```python
from build123d import *

# Parameters (mm, degrees)
F0_R     = 5.2
F0_R_2   = 2.5
F0_R_3   = 1.25
F0_R_4   = 3
F0_R_5   = 13
F1_DEPTH = 10
F2_DEPTH = 4


with BuildPart() as f1:
    # F0 (on Top) → F1 (new body)
    with BuildSketch(Plane.XY):
        with BuildLine():
            Line((-231, -59.5), (231, -59.5))
            ThreePointArc((231, -59.5), (235.242641, -57.742641), (237, -53.5))
            Line((237, -53.5), (237, 53.5))
            ThreePointArc((237, 53.5), (235.242641, 57.742641), (231, 59.5))
            Line((231, 59.5), (-231, 59.5))
            ThreePointArc((-231, 59.5), (-235.242641, 57.742641), (-237, 53.5))
            Line((-237, 53.5), (-237, -53.5))
            ThreePointArc((-237, -53.5), (-235.242641, -57.742641), (-231, -59.5))
        make_face()
        with Locations((-217, -39.5)):
            Circle(F0_R, mode=Mode.SUBTRACT)
        with Locations((-81, -13.5)):
            Circle(F0_R_2, mode=Mode.SUBTRACT)
        with Locations((-66, -13.5)):
            Circle(F0_R_2, mode=Mode.SUBTRACT)
        with Locations((-81, -4)):
            Circle(F0_R_3, mode=Mode.SUBTRACT)
        with Locations((-53, -13.5)):
            Circle(F0_R_4, mode=Mode.SUBTRACT)
        with Locations((0, -13.5)):
            Circle(F0_R_5, mode=Mode.SUBTRACT)
        with Locations((217, -39.5)):
            Circle(F0_R, mode=Mode.SUBTRACT)
        with Locations((29, -13.5)):
            Circle(F0_R_2, mode=Mode.SUBTRACT)
        with Locations((42, -13.5)):
            Circle(F0_R_2, mode=Mode.SUBTRACT)
        with Locations((55, -13.5)):
            Circle(F0_R_2, mode=Mode.SUBTRACT)
        with Locations((68, -13.5)):
            Circle(F0_R_2, mode=Mode.SUBTRACT)
        with Locations((81, -13.5)):
            Circle(F0_R_2, mode=Mode.SUBTRACT)
        with BuildLine():
            ThreePointArc((-198, 31.5), (-196.828427, 34.328427), (-194, 35.5))
            Line((-194, 35.5), (-115, 35.5))
            ThreePointArc((-115, 35.5), (-112.171573, 34.328427), (-111, 31.5))
            Line((-111, 31.5), (-111, -23.5))
            ThreePointArc((-111, -23.5), (-112.171573, -26.328427), (-115, -27.5))
            Line((-115, -27.5), (-194, -27.5))
            ThreePointArc((-194, -27.5), (-196.828427, -26.328427), (-198, -23.5))
            Line((-198, -23.5), (-198, 31.5))
        make_face(mode=Mode.SUBTRACT)
        with BuildLine():
            Line((-79, 35.5), (79, 35.5))
            ThreePointArc((79, 35.5), (81.828427, 34.328427), (83, 31.5))
            Line((83, 31.5), (83, 9.5))
            ThreePointArc((83, 9.5), (81.828427, 6.671573), (79, 5.5))
            Line((79, 5.5), (-79, 5.5))
            ThreePointArc((-79, 5.5), (-81.828427, 6.671573), (-83, 9.5))
            Line((-83, 9.5), (-83, 31.5))
            ThreePointArc((-83, 31.5), (-81.828427, 34.328427), (-79, 35.5))
        make_face(mode=Mode.SUBTRACT)
        with Locations((-217, 39.5)):
            Circle(F0_R, mode=Mode.SUBTRACT)
        with BuildLine():
            Line((111, -23.5), (111, 31.5))
            ThreePointArc((111, 31.5), (112.171573, 34.328427), (115, 35.5))
            Line((115, 35.5), (194, 35.5))
            ThreePointArc((194, 35.5), (196.828427, 34.328427), (198, 31.5))
            Line((198, 31.5), (198, -23.5))
            ThreePointArc((198, -23.5), (196.828427, -26.328427), (194, -27.5))
            Line((194, -27.5), (115, -27.5))
            ThreePointArc((115, -27.5), (112.171573, -26.328427), (111, -23.5))
        make_face(mode=Mode.SUBTRACT)
        with Locations((217, 39.5)):
            Circle(F0_R, mode=Mode.SUBTRACT)
    extrude(amount=F1_DEPTH)

    # F0 (on Top) → F2 (join)
    with BuildSketch(Plane.XY):
        with Locations((-217, 39.5)):
            Circle(F0_R)
        with Locations((-217, 39.5)):
            Circle(F0_R_4, mode=Mode.SUBTRACT)
        with Locations((-217, -39.5)):
            Circle(F0_R)
        with Locations((-217, -39.5)):
            Circle(F0_R_4, mode=Mode.SUBTRACT)
        with Locations((217, -39.5)):
            Circle(F0_R)
        with Locations((217, -39.5)):
            Circle(F0_R_4, mode=Mode.SUBTRACT)
        with Locations((217, 39.5)):
            Circle(F0_R)
        with Locations((217, 39.5)):
            Circle(F0_R_4, mode=Mode.SUBTRACT)
    extrude(amount=F2_DEPTH)


solid = f1.part
```
Input: part model. Units: mm. Frame: model coordinates. A direction names the side the tool comes from. Round coordinates to 2 decimals unless told otherwise and drop trailing zeros. Write each loop counter-clockwise with the first axis right and the second up, starting at its lowest first coordinate (ties: lowest second). Pieces come first, ordered by that corner, then holes. Notation, with made-up numbers: M 20.25,7 L 34.25,7 A9 ccw 34.25,22 Z; hole C 16,-7.75 d1. An arc over 180 degrees is marked long. Write each question's results on one line, items separated by ' | '.
Q1. Section query A-A (x = 186). Return loops of the section in (y, z).
Results:
outline: M -59.5,0 L -27.5,0 L -27.5,10 L -59.5,10 Z; M 35.5,0 L 59.5,0 L 59.5,10 L 35.5,10 Z
Q2. Draft query along Y for faces 4 (the face through (3, 59.5, 5)), 5 (the face through (-237, 1, 5)), 6 (the face through (221.96, 41.06, 6.96)), 7 (the face through (-3, -59.5, 5)). Return one class per face: released by +Y, released by -Y, zero draft, split by the parting line, or undercut.
Results:
face 4: released by +Y | face 5: zero draft | face 6: undercut | face 7: released by -Y
Q3. Section query C-C (z = 1.5). State how many separate pieces and enclosed holes the cut face has, and give its area (3 significant figures).
Results:
separate pieces: 1 | enclosed holes: 17 | area: 39,700 mm^2
Q4. Line query: line 1 along Y through (x, z) = (217, 8.2); line 2 along X through (y, z) = (25, 9); line 3 along Y through (x, z) = (55, 7.5). Output: solid intervals per line, ascending.
Results:
line 1: y = -59.5 to -44.7, -34.3 to 34.3, 44.7 to 59.5 | line 2: x = -237 to -198, -111 to -83, 83 to 111, 198 to 237 | line 3: y = -59.5 to -16, -11 to 5.5, 35.5 to 59.5
Q5. Access query for faces 1 (the face through (237, -1, 5)), 2 (the face through (-154, -27.5, 5)), 3 (the face through (219, -42, 4)). Directions: +Z, -Z, +X, -X, +Y, -Y. A direction counts if a zero-diameter tool reaches every point of the face in a straight line with its end or side. Return the directions, or none.
Results:
face 1: +Z, -Z, +X, +Y, -Y | face 2: +Z, -Z | face 3: +Z
Q6. Section query B-B (y = 20.5). Return loops of the section in (x, z), and give its area (3 significant figures).
Results:
outline: M -237,0 L -198,0 L -198,10 L -237,10 Z; M -111,0 L -83,0 L -83,10 L -111,10 Z; M 83,0 L 111,0 L 111,10 L 83,10 Z; M 198,0 L 237,0 L 237,10 L 198,10 Z | area: 1,340 mm^2
Q7. Pin query (flat end, axial travel): P1, Ø3, axis at x = 81, y = -13.5, coming from the -Z side; P2, Ø5, axis at x = 214.5, y = 39, coming from the +Z side. Return the tip coordinate at first contact, or that it passes through.
Results:
P1: passes through | P2: stops at z = 4
